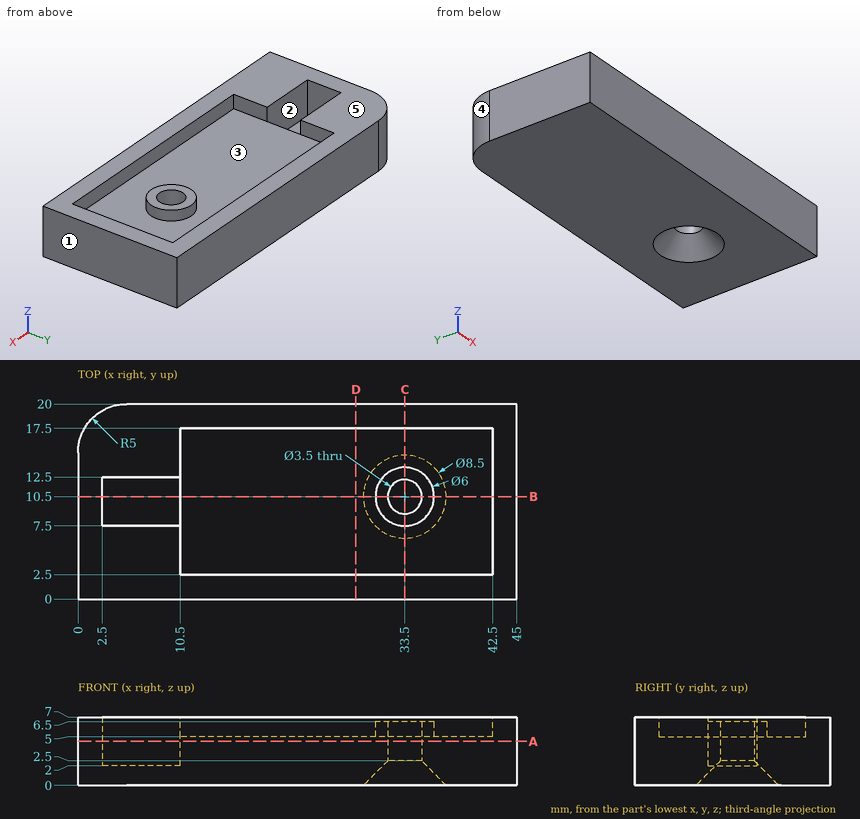
Part print with two shaded views. Sizes in mm from the minimum x, y, z corner. A direction names the side the tool comes from. Round coordinates to 2 decimals unless told otherwise and drop trailing zeros. Write each loop counter-clockwise with the first axis right and the second up, starting at its lowest first coordinate (ties: lowest second). Pieces come first, ordered by that corner, then holes. Notation, with made-up numbers: M 12,-39 L 50,-39 A29 cw 50,-7 Z; hole C 73,7.25 d6. An arc over 180 degrees is marked long. Answer as CSV lines item,"result". Start each with the question number.
1) Drop flat-ended pins along their axis: pin 1 (12 mm diameter, centred on x = 26, y = 9, fed in from +Z); pin 2 (1.5 mm diameter, centred on y = 3.5, z = 6, fed in from -X); pin 3 (2.5 mm diameter, centred on x = 8.5, y = 11, fed in from +Z). Give the stop position or say it passes through.
2) Band-saw the part on B-B (y = 10.5). List the corners of the cut face in (x, z), then the cut area to 3 significant figures.
3) Band-saw the part on A-A (z = 4.5). List the corners of the cut face in (x, y), then the cut area to 3 significant figures.
4) Which spindle directions (+Z, -Z, +X, -X, +Y, -Y) get a long thin tool onto all of the face, cutting with end or side? Do the marked faces 1 and 2. Say none if no direction does.
5) Band-saw the part on D-D (x = 28.5). List the corners of the cut face in (y, z).
6) Mould opens along X. For the marked faces 3, 4 and 5 say: +X half, -X half, draft (parallel to the pull), parting line (faces both ways), or undercut.
7) Band-saw the part on C-C (x = 33.5). List the corners of the cut face in (y, z), then the cut area to 3 significant figures.
8) Drill centre lines: L1, parallel to Y at x = 33.5, z = 5.1; L2, parallel to Y at x = 7.5, z = 2.75; L3, parallel to Y at x = 33.5, z = 3.75. Where is each one in solid material? Low to high.
Worked out:
1,pin 1,"z = 6.5"
1,pin 2,"x = 0"
1,pin 3,"z = 2"
2,outline,"M 0,0 L 29.25,0 L 31.75,2.5 L 31.75,6.5 L 30.5,6.5 L 30.5,5 L 10.5,5 L 10.5,2 L 2.5,2 L 2.5,7 L 0,7 Z; M 35.25,2.5 L 37.75,0 L 45,0 L 45,7 L 42.5,7 L 42.5,5 L 36.5,5 L 36.5,6.5 L 35.25,6.5 Z"
2,area,"191 mm²"
3,outline,"M 0,0 L 45,0 L 45,20 L 5,20 A5 ccw 0,15 Z; hole M 2.5,7.5 L 10.5,7.5 L 10.5,12.5 L 2.5,12.5 Z; hole C 33.5,10.5 d3.5"
3,area,"845 mm²"
4,face 1,"+Z, -Z, +X, +Y, -Y"
4,face 2,"+Z"
5,outline,"M 0,0 L 20,0 L 20,7 L 17.5,7 L 17.5,5 L 2.5,5 L 2.5,7 L 0,7 Z"
6,face 3,"undercut"
6,face 4,"-X half"
6,face 5,"draft"
7,outline,"M 0,0 L 6.25,0 L 8.75,2.5 L 8.75,6.5 L 7.5,6.5 L 7.5,5 L 2.5,5 L 2.5,7 L 0,7 Z; M 12.25,2.5 L 14.75,0 L 20,0 L 20,7 L 17.5,7 L 17.5,5 L 13.5,5 L 13.5,6.5 L 12.25,6.5 Z"
7,area,"90.0 mm²"
8,L1,"0 to 2.5, 7.5 to 8.75, 12.25 to 13.5, 17.5 to 20"
8,L2,"0 to 7.5, 12.5 to 20"
8,L3,"0 to 8.75, 12.25 to 20"
